```python
from build123d import *

# Parameters (mm, degrees)
CROQUIS1_W              = 90.62
CROQUIS1_H              = 65.8
CROQUIS1_R              = 1.5
SALIENTE_EXTRUIR1_DEPTH = 3
CROQUIS2_W              = 22.5
CROQUIS2_H              = 15
SALIENTE_EXTRUIR2_DEPTH = 1


with BuildPart() as part:
    # Croquis1 → Saliente-Extruir1 (new body)
    with BuildSketch(Plane(origin=(0, 0, 0), x_dir=(0, 0, -1), z_dir=(1, 0, 0))):
        with Locations((45.31, 32.9)):
            Rectangle(CROQUIS1_W, CROQUIS1_H)
        with Locations((88.12, 63.3)):
            Circle(CROQUIS1_R, mode=Mode.SUBTRACT)
        with Locations((87.12, 3.5)):
            Circle(CROQUIS1_R, mode=Mode.SUBTRACT)
        with Locations((2.5, 3.5)):
            Circle(CROQUIS1_R, mode=Mode.SUBTRACT)
    extrude(amount=SALIENTE_EXTRUIR1_DEPTH)

    # Croquis2 → Saliente-Extruir2 (add)
    with BuildSketch(Plane(origin=(3, 0, 0), x_dir=(0, 0, -1), z_dir=(1, 0, 0))):
        with Locations((59.37, 32.3)):
            Rectangle(CROQUIS2_W, CROQUIS2_H)
    extrude(amount=SALIENTE_EXTRUIR2_DEPTH)


solid = part.part
```
Read the model definition and answer for the solid it produces. Units are mm, in the model's axes. Round coordinates to 2 decimals unless told otherwise and drop trailing zeros. Write each loop counter-clockwise with the first axis right and the second up, starting at its lowest first coordinate (ties: lowest second). Pieces come first, ordered by that corner, then holes. Notation, with made-up numbers: M -24,3 L -13,3 A10 ccw -13,9 Z; hole C 80.25,-32.75 d2. An arc over 180 degrees is marked long. One line per item, written item: value.
Q1. For a pull along Y with two mould halves and no side action, classify faces 1 (the cylindrical face through (1.48, 3.57, -85.62)), 2 (the flat face through (0, 33, -45)), 3 (the flat face through (1, 0, -45)) as +Y half, -Y half, draft (parallel to the pull), parting line (faces both ways), or undercut.
Data:
face 1: undercut
face 2: draft
face 3: -Y half
Q2. Find section A-A on z = -2.5. Write down the section's boundary in (x, y).
Data:
outline: M 0,0 L 3,0 L 3,2 L 0,2 Z; M 0,5 L 3,5 L 3,65.8 L 0,65.8 Z
Q3. Straight lines are drawn through the part: line 1 (Y direction, x = 1.6, z = -2.5); line 2 (Y direction, x = 1.95, z = -88.12); line 3 (X direction, y = 23.5, z = -84). For each, find the intervals that lie inside material, in ascending order. Write a range as [from, to].
Data:
line 1: [0, 2], [5, 65.8]
line 2: [0, 2.38], [4.62, 61.8], [64.8, 65.8]
line 3: [0, 3]
Q4. Find section B-B on y = 3.5. Write down the section's boundary in (x, z).
Data:
outline: M 0,-90.62 L 3,-90.62 L 3,-88.62 L 0,-88.62 Z; M 0,-85.62 L 3,-85.62 L 3,-4 L 0,-4 Z; M 0,-1 L 3,-1 L 3,0 L 0,0 Z
Q5. Flat-ended cylindrical pins translate along their axes: pin 1 Ø0.5 at (x, z) = (3.5, -58.5) entering from -Y; pin 2 Ø0.8 at (x, y) = (3.5, 33.5) entering from +Z; pin 3 Ø8 at (y, z) = (6.5, -63) entering from +X. Find the tip coordinate at first contact, or state that the pin passes through.
Data:
pin 1: y = 24.8
pin 2: z = -48.12
pin 3: x = 3
Q6. Find section D-D on z = -52. Write down the section's boundary in (x, y), plus the area to 3 significant figures.
Data:
outline: M 0,0 L 3,0 L 3,24.8 L 4,24.8 L 4,39.8 L 3,39.8 L 3,65.8 L 0,65.8 Z
area: 212 mm2
Q7. Find section C-C on y = 63.3. Write down the section's boundary in (x, z).
Data:
outline: M 0,-90.62 L 3,-90.62 L 3,-89.62 L 0,-89.62 Z; M 0,-86.62 L 3,-86.62 L 3,0 L 0,0 Z
